The listing builds one solid part. Answer for the finished solid, in the listing's coordinates (mm). Face numbers are marked on the shaded views. A direction names the side the tool comes from. Coordinates: 2 decimals unless noted, no trailing zeros. Order: outer loops, then holes, each group sorted by start corner. A loop starts at its lowest first (then second) coordinate and runs counter-clockwise, first axis right, second up. Notation, with made-up numbers: (35.25, 1) -> (54.25, 1) arc R15 ccw to (54.25, 22) -> close; hole circle Ø2 at (52.5, 29.5). An arc over 180 degrees is marked (long way). Write item = value, one per line.
from build123d import *

# Parameters (mm, degrees)
SKETCH_1_R          = 15.85
EXTRUDE_1_DEPTH     = 12
SKETCH_2_R          = 10.1
CUT_EXTRUDE_1_DEPTH = 2.5
SKETCH_3_R          = 11
CUT_EXTRUDE_2_DEPTH = 7.5
SKETCH_4_R          = 1.5
CUT_EXTRUDE_3_DEPTH = 6
EXTRUDE_2_DEPTH     = 1
SKETCH_7_R          = 1
CUT_EXTRUDE_4_DEPTH = 16


with BuildPart() as part:
    # 草图1 → 凸台-拉伸1 (new body)
    with BuildSketch(Plane(origin=(0, 0, 0), x_dir=(1, 0, 0), z_dir=(0, 1, 0))):
        with Locations(Location((0, 0, 0), (0, 0, 270))):
            Circle(SKETCH_1_R)
    extrude(amount=EXTRUDE_1_DEPTH)

    # 草图2 → 切除-拉伸1 (cut)
    with BuildSketch(Plane.XZ):
        with Locations(Location((0, 0, 0), (0, 0, 270))):
            Circle(SKETCH_2_R)
    extrude(amount=-CUT_EXTRUDE_1_DEPTH, mode=Mode.SUBTRACT)

    # 草图3 → 切除-拉伸2 (cut)
    with BuildSketch(Plane(origin=(0, 12, 0), x_dir=(1, 0, 0), z_dir=(0, 1, 0))):
        with Locations(Location((0, 0, 0), (0, 0, 270))):
            Circle(SKETCH_3_R)
    extrude(amount=-CUT_EXTRUDE_2_DEPTH, mode=Mode.SUBTRACT)

    # 草图4 → 切除-拉伸3 (cut)
    with BuildSketch(Plane.XZ.offset(-2.5)):
        with Locations(Location((0, 7, 0), (0, 0, 270))):
            Circle(SKETCH_4_R)
        with Locations(Location((7, 0, 0), (0, 0, 270))):
            Circle(SKETCH_4_R)
        with Locations(Location((0, -7, 0), (0, 0, 270))):
            Circle(SKETCH_4_R)
        with Locations(Location((-7, 0, 0), (0, 0, 270))):
            Circle(SKETCH_4_R)
        with Locations(Location((0, 0, 0), (0, 0, 270))):
            Circle(SKETCH_4_R)
    extrude(amount=-CUT_EXTRUDE_3_DEPTH, mode=Mode.SUBTRACT)

    # 草图5 → 切除-旋转1 (revolve, cut)
    with BuildSketch(Plane(origin=(0, 0, 0), x_dir=(0, 0, -1), z_dir=(1, 0, 0)), mode=Mode.PRIVATE) as cut_revolve_1_sk:
        Polygon((-15.35, 11), (-12.6, 9.41228676), (-12.6, 0), (-15.85, 0), (-15.85, 11), align=None)
    revolve(cut_revolve_1_sk.sketch.rotate(Axis((0, -0.5, 0), (0, 1, 0)), 180), axis=Axis((0, -0.5, 0), (0, 1, 0)), mode=Mode.SUBTRACT)

    # 草图6 → 凸台-拉伸2 (add)
    with BuildSketch(Plane(origin=(0, 4, 0), x_dir=(1, 0, 0), z_dir=(0, 1, 0))):
        with BuildLine():
            Line((11.485757101, 4.932279778), (12.297768749, 4.932279778))
            ThreePointArc((12.297768749, 4.932279778), (-13.25, 0), (12.297768749, -4.932279778))
            Line((12.297768749, -4.932279778), (11.485757101, -4.932279778))
            ThreePointArc((11.485757101, -4.932279778), (-12.5, 0), (11.485757101, 4.932279778))
        make_face()
    extrude(amount=EXTRUDE_2_DEPTH)

    # 草图7 → 切除-拉伸4 (cut)
    with BuildSketch(Plane(origin=(0, 0, 0), x_dir=(0, 0, -1), z_dir=(1, 0, 0))):
        with Locations((0, 6)):
            Circle(SKETCH_7_R)
    extrude(amount=-CUT_EXTRUDE_4_DEPTH, mode=Mode.SUBTRACT)


solid = part.part
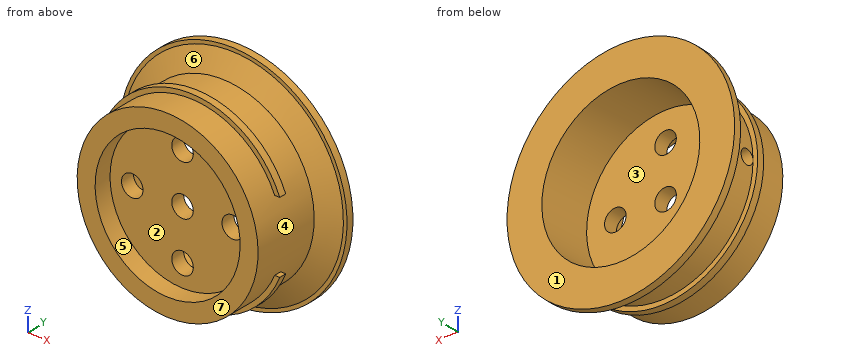
Q1. Section C-C, the plane y = 5.5 is taken. Give the vertices of the cut face in (x, z).
The answers:
outline = (-12.57, -0.87) arc R12.6 ccw (long way) to (-12.57, 0.87) -> (-10.97, 0.87) arc R11 cw (long way) to (-10.97, -0.87) -> close
Q2. Section B-B, the plane x = 0 is taken. Give the number of separate pieces and of enclosed holes in the cut face, plus the area to 3 significant figures.
The answers:
separate_pieces = 4
enclosed_holes = 0
area = 81.1 mm2
Q3. Each of these flat-tipped pins is pushed along its axis until it touches: pin 1 Ø5 at (x, z) = (-7, 0) entering from +Y; pin 2 Ø0.8 at (x, y) = (12, 4.5) entering from +Z; pin 3 Ø3.5 at (x, z) = (7, 0) entering from -Y. Where does it stop, or does it pass through?
The answers:
pin_1 = 4.5
pin_2 = 6.4
pin_3 = 2.5
Q4. Find the intervals of material crossed by line 1 along X through (y, z) = (4.05, 0); line 2 along X through (y, z) = (3.75, 0); line 3 along Y through (x, z) = (3, -5.5), in increasing order.
The answers:
line_1 = -13.25 to -8.5, -5.5 to -1.5, 1.5 to 5.5, 8.5 to 12.6
line_2 = -12.6 to -8.5, -5.5 to -1.5, 1.5 to 5.5, 8.5 to 12.6
line_3 = 2.5 to 4.5
Q5. The mould has two halves that part along Z. Classify the marked faces 5, 6 and 7: released by +Z, released by -Z, zero draft, split by the parting line, or undercut.
The answers:
face_5 = undercut
face_6 = split by the parting line
face_7 = zero draft
Q6. Section A-A, the plane y = 3 is taken. Give the vertices of the cut face in (x, z), plus the area to 3 significant figures.
The answers:
outline = circle Ø25.2 at (0, 0); hole circle Ø3 at (-7, 0); hole circle Ø3 at (0, -7); hole circle Ø3 at (0, 0); hole circle Ø3 at (0, 7); hole circle Ø3 at (7, 0)
area = 463 mm2
Q7. A tool of negligible diameter and unlimited length cuts with its end or side. For the marked faces 1, 2, 3 and 4, from which of +Z, -Z, +X, -X, +Y, -Y can it reach the whole face along a straight path? Write none if from no direction.
The answers:
face_1 = +Z, -Z, +X, -X, +Y
face_2 = -Y
face_3 = +Y
face_4 = none
